Read the model definition and answer for the solid it produces. Units are mm, in the model's axes. Face numbers are marked on the shaded views. A direction names the side the tool comes from. Coordinates: 2 decimals unless noted, no trailing zeros. Loops run counter-clockwise (first coordinate to the right, second up) from the corner with the lowest first, then second, coordinate; pieces in that order, holes last. Notation, with made-up numbers: (57.5, 56.5) - (83.5, 56.5) arc R33 cw to (83.5, 90.5) - close; hole circle Ø1 at (40.25, 74). An arc over 180 degrees is marked (long way). Use one line per item in the form item = value. Start each with the question number.
1) A cutting plane is placed at B-B (x = 128). Give the vertices of the cut face in (y, z).
2) A cutting plane is placed at A-A (y = 122). Give the vertices of the cut face in (x, z), and give its area (3 significant figures).
3) A cutting plane is placed at C-C (y = 47). Give the vertices of the cut face in (x, z).
4) A cutting plane is placed at D-D (x = 91). Give the vertices of the cut face in (y, z).
5) Each of these flat-tipped pins is pushed along its axis until it touches: P1, Ø6, axis at x = 116, y = 125, coming from the +Z side; P2, Ø2, axis at y = 113, z = 1.5, coming from the +X side; P3, Ø4, axis at y = 20, z = -4, coming from the +X side; P4, Ø1.6, axis at y = 40, z = 0.5, coming from the +X side. Where does it stop, or does it pass through?
6) Consider line 1 (Y direction, x = 120.5, z = 0.75); line 2 (Y direction, x = 60, z = 0.4); line 3 (X direction, y = 40, z = 1.1). Determine where each line is inside the solid, lowest interval first.
7) Which of the six approach directions +Z, -Z, +X, -X, +Y, -Y give full straight-line access (tool end or side, diameter ignored) to the marked faces 1 and 2?
Autodesk Inventor part; units mm, degrees
ref_plane "YZ Plane" through (0, 0, 0) normal (1, 0, 0) x (0, 1, 0)
ref_plane "XZ Plane" through (0, 0, 0) normal (0, 1, 0) x (-1, 0, 0)
ref_plane "XY Plane" through (0, 0, 0) normal (0, 0, 1) x (1, 0, 0)
sketch "Sketch1" plane through (0, 0, 0) normal (0, 0, 1) x (1, 0, 0)
  line L0 (0, 0) -> (260, 0)
  line L1 (260, 0) -> (260, 125)
  line L2 (220, 147) -> (0, 147)
  line L3 (0, 147) -> (0, 0)
  circle A0 centre (240, 135) radius 8
  circle A1 centre (240, 135) radius 10
  line L4 (250, 135) -> (250.202, 135)
  line L5 (230, 135) -> (230, 137)
  arc A2 (230, 137) -> (220, 147) centre (220, 137) ccw
  line L6 (260, 147) -> (260, 147)
  line L7 (250, 135) -> (250, 137)
  line L8 (240, 125) -> (260, 125)
  line L9 (0, 73.5) -> (260, 73.5)
  line L10 (130, 112.7628) -> (117.7684, 112.7628)
  line L11 (99.8322, 119.3312) -> (99.8322, 90.3139)
  line L12 (99.8322, 90.3139) -> (148.259, 90.3139)
  line L13 (148.259, 90.3139) -> (148.259, 44.839)
  line L14 (148.259, 44.839) -> (117.7684, 44.839)
  line L15 (99.8322, 44.839) -> (99.8322, 25.7829)
  line L16 (99.8322, 25.7829) -> (130, 25.7829)
  line L17 (99.8322, 119.3312) -> (99.8322, 127)
  line L18 (99.8322, 127) -> (117.7684, 127)
  line L19 (117.7684, 127) -> (117.7684, 112.7628)
  line L20 (99.8322, 44.839) -> (99.8322, 55.475)
  line L21 (99.8322, 55.475) -> (117.7684, 55.475)
  line L22 (117.7684, 55.475) -> (117.7684, 44.839)
  line L23 (130, 147) -> (130, 112.7628)
  line L24 (130, 25.7829) -> (130, 0)
  line L25 (60, 107) -> (200, 107)
  line L26 (200, 107) -> (200, 40)
  line L27 (200, 40) -> (60, 40)
  line L28 (60, 40) -> (60, 107)
  circle A3 centre (60, 107) radius 1.5
  circle A4 centre (200, 107) radius 1.5
  circle A5 centre (200, 40) radius 1.5
  circle A6 centre (60, 40) radius 1.5
  circle A7 centre (130, 107) radius 1.5
  circle A8 centre (130, 40) radius 1.5
  line L29 (260, 125) -> (265, 125)
  line L30 (265, 0) -> (260, 0)
  line L31 (260, 0) -> (260, 125)
  line L32 (265, 0) -> (263, 0)
  line L33 (0, 147) -> (-3, 147)
  line L34 (-3, 147) -> (-3, 0)
  line L35 (-3, 0) -> (0, 0)
  line L36 (0, 0) -> (0, 147)
  line L37 (-3, 147) -> (-5, 147)
  line L38 (-5, 147) -> (-5, 0)
  line L39 (-5, 0) -> (-3, 0)
  line L40 (-3, 0) -> (-3, 147)
  point P0 (260, 67.5)
  point P1 (263, 125)
  point P2 (200, 73.5)
  point P3 (148.259, 73.5)
  point P4 (99.8322, 107)
  point P5 (128.5, 107)
  point P6 (131.5, 107)
  point P7 (198.5, 107)
  point P8 (200, 105.5)
  point P9 (60, 73.5)
  point P10 (99.8322, 40)
  dimension "d2" = 16
  dimension "d3" = 20
  dimension "d4" = 135
  dimension "d5" = 2
  dimension "d6" = 260
  dimension "d7" = 147
  dimension "d8" = 10
  dimension "d11" = 22
  dimension "d16" = 40
  dimension "d17" = 40
  dimension "d18" = 60
  dimension "d19" = 60
  dimension "d20" = 3
  dimension "d21" = 3
  dimension "d22" = 3
  dimension "d23" = 3
  dimension "d24" = 140
  dimension "d25" = 67
  dimension "d26" = 3
  dimension "d27" = 3
  dimension "d28" = 70
  dimension "d29" = 70
  dimension "d30" = 5
  dimension "d31" = 2
  dimension "d41" = 3
  dimension "d42" = 2
extrude "Extrusion1" add sketch "Sketch1" along normal blind 2 contours L3 L9 L28 A6 L27 L15 L16 L24 L0 | L35 L34 L33 L3 | L3 L2 L23 L10 L19 L18 L17 L11 L25 A3 L28 L9 | L39 L38 L37 L34 | L28 A3 L25 L11 L12 L13 L9 | L9 L13 L14 L22 L21 L20 L15 L27 A6 L28
sketch "Sketch4" plane through (0, 0, 0) normal (0, 0, -1) x (-1, 0, 0)
  line L0 (-130, 147) -> (5, 147)
  line L1 (5, 0) -> (-130, 0)
  line L2 (5, 147) -> (3, 147)
  line L3 (3, 147) -> (3, 0)
  line L4 (3, 0) -> (5, 0)
  line L5 (5, 0) -> (5, 147)
  point P0 (0, 0)
  dimension "d43" = 2
extrude "Extrusion4" add sketch "Sketch4" along normal blind 10
sketch "Sketch5" plane through (-5, 0, 2) normal (-1, 0, 0) x (0, 0, 1)
  line L0 (-12, 147) -> (-12, 0)
  line L1 (-2, 0) -> (-12, 0)
  line L2 (-12, 147) -> (-6, 147)
  line L3 (-6, 147) -> (-6, 0)
  line L4 (-6, 0) -> (-12, 0)
  line L5 (-12, 0) -> (-12, 147)
  circle A0 centre (-6, 127) radius 1.5
  circle A1 centre (-6, 20) radius 1.5
  line L6 (-12, 147) -> (0, 147)
  line L7 (-12, 0) -> (0, 0)
  point P0 (-6, 147)
  point P1 (-6, 0)
  dimension "d46" = 6
  dimension "d47" = 3
  dimension "d48" = 3
  dimension "d49" = 20
  dimension "d50" = 20
extrude "Extrusion5" cut sketch "Sketch5" against normal blind 10 contours A0 L3 | L3 A0 | A1 L3 | L3 A1
properties part number "Coffee_Machine_Base"
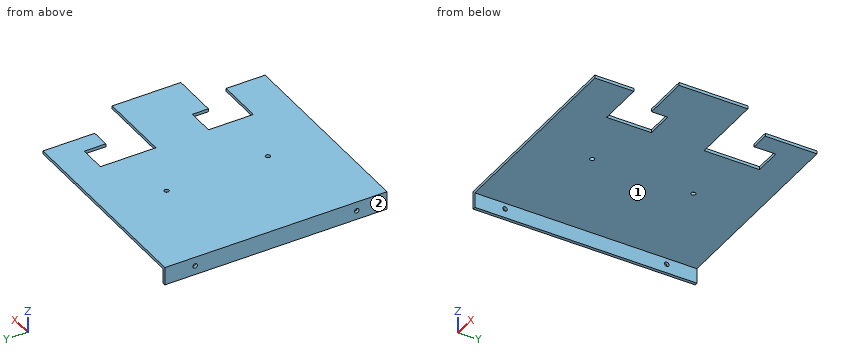
Found:
q1.outline = (0, 0) - (25.78, 0) - (25.78, 2) - (0, 2) - close; (44.84, 0) - (90.31, 0) - (90.31, 2) - (44.84, 2) - close; (112.76, 0) - (147, 0) - (147, 2) - (112.76, 2) - close
q2.outline = (-5, -10) - (-3, -10) - (-3, 0) - (99.83, 0) - (99.83, 2) - (-5, 2) - close; (117.77, 0) - (130, 0) - (130, 2) - (117.77, 2) - close
q2.area = 254 mm^2
q3.outline = (-5, -10) - (-3, -10) - (-3, 0) - (99.83, 0) - (99.83, 2) - (-5, 2) - close; (117.77, 0) - (148.26, 0) - (148.26, 2) - (117.77, 2) - close
q4.outline = (0, 0) - (147, 0) - (147, 2) - (0, 2) - close
q5.P1 = 2
q5.P2 = 130
q5.P3 = -3
q5.P4 = 99.83
q6.line_1 = 0 to 25.78, 44.84 to 90.31, 112.76 to 147
q6.line_2 = 0 to 38.5, 41.5 to 105.5, 108.5 to 147
q6.line_3 = -5 to 58.5, 61.5 to 99.83
q7.face_1 = -Z, +X, +Y, -Y
q7.face_2 = +Z, -Z, -X, +Y, -Y
